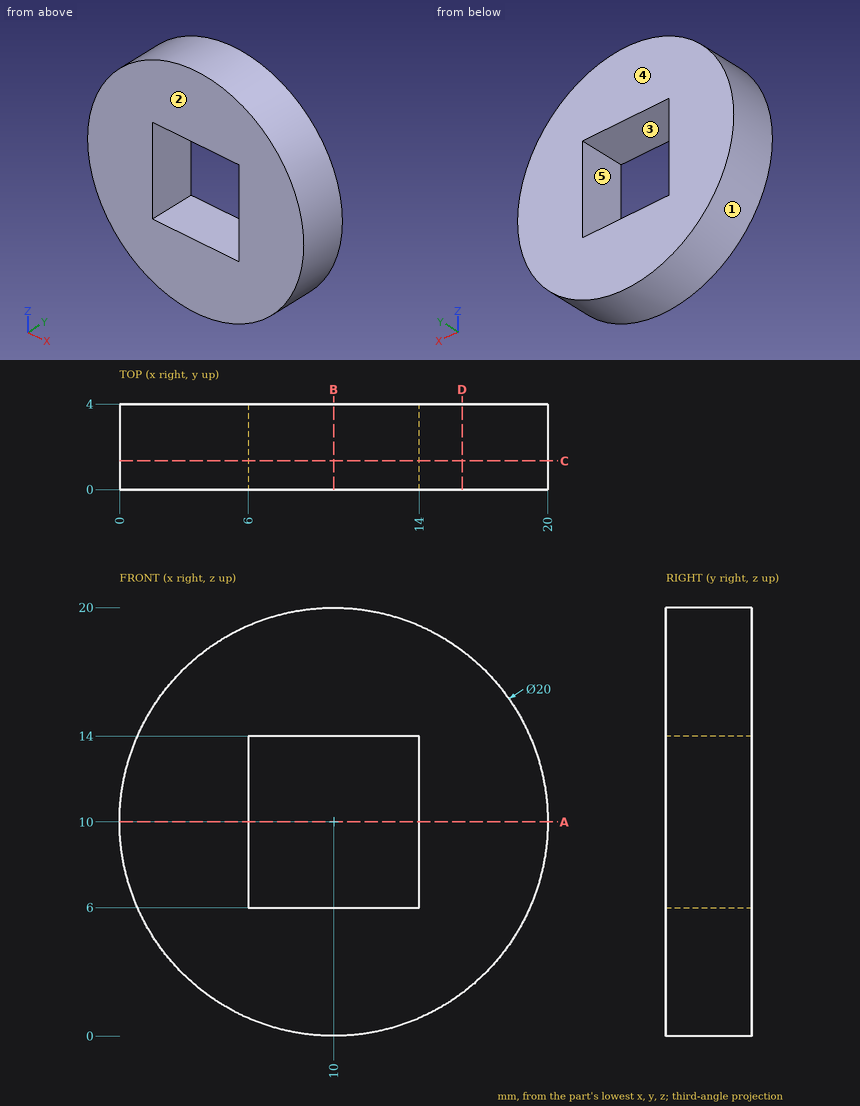
Answer from the drawing. Dimensions are ordinates in mm from the lowest x, y and z of the part. A direction names the side the tool comes from. Coordinates: 2 decimals unless noted, no trailing zeros. Write each loop counter-clockwise with the first axis right and the second up, starting at its lowest first coordinate (ties: lowest second). Pieces come first, ordered by that corner, then holes. Notation, with made-up numbers: M 87.25,-0.75 L 110.25,-0.75 A19 cw 110.25,25.25 Z; hole C 29.5,-3 d11. An arc over 180 degrees is marked long. Write item = value, one per line.
1. Flat-ended cylindrical pins translate along their axes: pin 1 (1 mm diameter, centred on x = 7.5, y = 1, fed in from +Z); pin 2 (1.2 mm diameter, centred on y = 2, z = 11.5, fed in from -X); pin 3 (2 mm diameter, centred on y = 1.5, z = 17.5, fed in from +X); pin 4 (3 mm diameter, centred on x = 7, z = 7, fed in from -Y). Find the tip coordinate at first contact, or state that the pin passes through.
Solution:
pin_1 = 19.8
pin_2 = 0.04
pin_3 = 17.6
pin_4 = 0
2. The part is cut by section C-C (y = 1.35). Determine the outline of the cut face in (x, z).
Solution:
outline = C 10,10 d20; hole M 6,6 L 14,6 L 14,14 L 6,14 Z
3. The part is cut by section B-B (x = 10). Determine the outline of the cut face in (y, z), then the cut area to 3 significant figures.
Solution:
outline = M 0,0 L 4,0 L 4,6 L 0,6 Z; M 0,14 L 4,14 L 4,20 L 0,20 Z
area = 48.0 mm2
4. Straight lines are drawn through the part: line 1 (X direction, y = 1.4, z = 7); line 2 (X direction, y = 3.3, z = 8); line 3 (Z direction, x = 12.75, y = 1.05). For each, find the intervals that lie inside material, in ascending order. Write a range as from..to.
Solution:
line_1 = 0.46..6, 14..19.54
line_2 = 0.2..6, 14..19.8
line_3 = 0.39..6, 14..19.61
5. For the marked faces 4 and 5, determine the directions among +Z, -Z, +X, -X, +Y, -Y from which every point of the face is accessible in a straight line to the end or side of a thin tool.
Solution:
face_4 = +Z, -Z, +X, -X, +Y
face_5 = +Y, -Y
6. Determine the mould class of the marked faces 1, 2 and 3 for opening direction X: released by +X, released by -X, zero draft, split by the parting line, or undercut.
Solution:
face_1 = split by the parting line
face_2 = zero draft
face_3 = undercut
7. The part is cut by section D-D (x = 16). Determine the outline of the cut face in (y, z).
Solution:
outline = M 0,2 L 4,2 L 4,18 L 0,18 Z
8. The part is cut by section A-A (z = 10). Determine the outline of the cut face in (x, y).
Solution:
outline = M 0,0 L 6,0 L 6,4 L 0,4 Z; M 14,0 L 20,0 L 20,4 L 14,4 Z
